from build123d import *

# Parameters (mm, degrees)
EXTRUDE_1_DEPTH = 1000


with BuildPart() as part:
    # Эскиз1 → Бобышка-Вытянуть1 (new body)
    with BuildSketch(Plane.XY):
        with BuildLine():
            Line((-4.1, 0), (-5, -0.158694283))
            Line((-5, -0.158694283), (-5, -0.8))
            Line((-5, -0.8), (-4.1, -0.8))
            Line((-4.1, -0.8), (-4.1, -4.196152423))
            Line((-4.1, -4.196152423), (-4.68771324, -5.214101615))
            Line((-4.68771324, -5.214101615), (-4.1, -6.232050808))
            ThreePointArc((-4.1, -6.232050808), (-3.497197677, -6.481739705), (-3.1, -5.964101615))
            Line((-3.1, -5.964101615), (-3.533012702, -5.214101615))
            Line((-3.533012702, -5.214101615), (-3.1, -4.464101615))
            Line((-3.1, -4.464101615), (-3.1, -1))
            Line((-3.1, -1), (3.1, -1))
            Line((3.1, -1), (3.1, -4.464101615))
            Line((3.1, -4.464101615), (3.533012702, -5.214101615))
            Line((3.533012702, -5.214101615), (3.1, -5.964101615))
            ThreePointArc((3.1, -5.964101615), (3.497197677, -6.481739705), (4.1, -6.232050808))
            Line((4.1, -6.232050808), (4.68771324, -5.214101615))
            Line((4.68771324, -5.214101615), (4.1, -4.196152423))
            Line((4.1, -4.196152423), (4.1, -0.8))
            Line((4.1, -0.8), (5, -0.8))
            Line((5, -0.8), (5, -0.158694283))
            Line((5, -0.158694283), (4.1, 0))
            Line((4.1, 0), (-4.1, 0))
        make_face()
    extrude(amount=EXTRUDE_1_DEPTH)


solid = part.part
Could you check a few things on this model? Use its own coordinates, in mm. Round coordinates to 2 decimals unless told otherwise and drop trailing zeros. Loops run counter-clockwise (first coordinate to the right, second up) from the corner with the lowest first, then second, coordinate; pieces in that order, holes last. Notation, with made-up numbers: (60.25, 65.5) -> (78.25, 65.5) arc R19 cw to (78.25, 69.5) -> close; hole circle Ø6 at (61.5, 54.5). An arc over 180 degrees is marked (long way). Use CSV: the item, a comma, the result in double quotes.
(1) Will these pins go through, and if not, where does the flat tip stop? pin 1 Ø1 at (x, z) = (0.5, 612) entering from +Y; pin 2 Ø3 at (y, z) = (-2.5, 371) entering from -X; pin 3 Ø3 at (x, z) = (1.5, 417) entering from -Y; pin 4 Ø1.5 at (y, z) = (-4, 340.5) entering from +X.
Return value:
pin 1,"stops at y = 0"
pin 2,"stops at x = -4.1"
pin 3,"stops at y = -1"
pin 4,"stops at x = 4.42"
(2) Suppose I cut it at B-B on z = 729. Write out the boundary of the cut face in (x, y).
Return value:
outline,"(-5, -0.8) -> (-4.1, -0.8) -> (-4.1, -4.2) -> (-4.69, -5.21) -> (-4.1, -6.23) arc R0.54 ccw to (-3.1, -5.96) -> (-3.53, -5.21) -> (-3.1, -4.46) -> (-3.1, -1) -> (3.1, -1) -> (3.1, -4.46) -> (3.53, -5.21) -> (3.1, -5.96) arc R0.54 ccw to (4.1, -6.23) -> (4.69, -5.21) -> (4.1, -4.2) -> (4.1, -0.8) -> (5, -0.8) -> (5, -0.16) -> (4.1, 0) -> (-4.1, 0) -> (-5, -0.16) -> close"
(3) If I drill on probe 1 along X at (y, z) = (-1.75, 746.5); probe 2 along Y at (x, z) = (-3.75, 96.5); probe 3 along Y at (x, z) = (-2.25, 691.5), over which ranges is the centre line in solid material (lowest first)? Write a range as [from, to].
Return value:
probe 1,"x = [-4.1, -3.1], [3.1, 4.1]"
probe 2,"y = [-6.49, 0]"
probe 3,"y = [-1, 0]"
(4) Suppose I cut it at C-C on x = 1.5. Write out the boundary of the cut face in (y, z).
Return value:
outline,"(-1, 0) -> (0, 0) -> (0, 1000) -> (-1, 1000) -> close"
(5) Suppose I cut it at A-A on y = -2.5. Write out the boundary of the cut face in (x, z), plus the area to 3 significant figures.
Return value:
outline,"(-4.1, 0) -> (-3.1, 0) -> (-3.1, 1000) -> (-4.1, 1000) -> close; (3.1, 0) -> (4.1, 0) -> (4.1, 1000) -> (3.1, 1000) -> close"
area,"2,000 mm²"
